```python
from build123d import *

# Parameters (mm, degrees)
SALIENTE_EXTRUIR1_DEPTH = 15
CROQUIS2_R              = 2.167600076
SALIENTE_EXTRUIR2_DEPTH = 1.2


with BuildPart() as part:
    # Croquis1 → Saliente-Extruir1 (new body)
    with BuildSketch(Plane.XY):
        Polygon((0, 0), (0, 10.369319961), (14.4, 10.369319961), (14.4, 0), (13.2, 0), (13.2, 8.869319961), (1.2, 8.869319961), (1.2, 0), align=None)
    extrude(amount=-SALIENTE_EXTRUIR1_DEPTH)

    # Croquis2 → Saliente-Extruir2 (add)
    # profile 1 of 2: a face of its own
    with BuildSketch(Plane.XZ):
        with BuildLine():
            ThreePointArc((20.704683633, -6.742646275), (24.235200152, -10.595528965), (20.704683633, -14.448411655))
            Line((20.704683633, -14.448411655), (14.4, -15))
            Line((14.4, -15), (14.4, -6.19105793))
            Line((14.4, -6.19105793), (20.704683633, -6.742646275))
        make_face()
        with Locations(Location((20.367600076, -10.595528965, 0), (0, 0, 270))):
            Circle(CROQUIS2_R, mode=Mode.SUBTRACT)
    # profile 2 of 2: a face of its own
    with BuildSketch(Plane.XZ):
        with BuildLine():
            Line((-6.304683633, -14.448411655), (0, -15))
            Line((0, -15), (0, -6.19105793))
            Line((0, -6.19105793), (-6.304683633, -6.742646275))
            ThreePointArc((-6.304683633, -6.742646275), (-9.835200152, -10.595528965), (-6.304683633, -14.448411655))
        make_face()
        with Locations(Location((-5.967600076, -10.595528965, 0), (0, 0, 270))):
            Circle(CROQUIS2_R, mode=Mode.SUBTRACT)
    extrude(amount=-SALIENTE_EXTRUIR2_DEPTH)


solid = part.part
```
Verification items for the finished model (mm, model axes). A direction names the side the tool comes from. Give positions to 0.01 mm unless a question says otherwise; leave off trailing zeros. Write each loop counter-clockwise with the first axis right and the second up, starting at its lowest first coordinate (ties: lowest second). Pieces come first, ordered by that corner, then holes. Notation, with made-up numbers: (58.5, 82.25) - (103.5, 82.25) arc R20 cw to (103.5, 103.25) - close; hole circle Ø11 at (54.5, 44.25). An arc over 180 degrees is marked (long way). Put each result on its own line as item: value.
Q1. Section check B-B on z = -10.25. Record the cut outline in (x, y), and give its area (3 significant figures).
Result:
outline: (-9.82, 0) - (-8.11, 0) - (-8.11, 1.2) - (-9.82, 1.2) - close; (-3.83, 0) - (1.2, 0) - (1.2, 8.87) - (13.2, 8.87) - (13.2, 0) - (18.23, 0) - (18.23, 1.2) - (14.4, 1.2) - (14.4, 10.37) - (0, 10.37) - (0, 1.2) - (-3.83, 1.2) - close; (22.51, 0) - (24.22, 0) - (24.22, 1.2) - (22.51, 1.2) - close
area: 56.2 mm2
Q2. Section check C-C on x = -5. Record the cut outline in (y, z), and give its area (3 significant figures).
Result:
outline: (0, -14.56) - (1.2, -14.56) - (1.2, -12.54) - (0, -12.54) - close; (0, -8.66) - (1.2, -8.66) - (1.2, -6.63) - (0, -6.63) - close
area: 4.87 mm2
Q3. Depth check by flat-ended pin: P1, Ø4.5, axis at x = 17.5, z = -11.5, coming from the +Y side; P2, Ø5, axis at y = 5, z = -6, coming from the -X side; P3, Ø5, axis at y = 8, z = -4.5, coming from the +X side. Enter the tip coordinate at first touch or a pass-through.
Result:
P1: y = 1.2
P2: x = 0
P3: x = 14.4
Q4. Scan lines: probe 1 along X at (y, z) = (7.25, -11.75); probe 2 along Y at (x, z) = (12, -13.25); probe 3 along X at (y, z) = (9.5, -13). Record each from-to range of solid material in increasing order. Write a range as from..to.
Result:
probe 1: 0..1.2, 13.2..14.4
probe 2: 8.87..10.37
probe 3: 0..14.4
Q5. Mould release check, pull along X, two halves, no side actions. Record for faces 5 (the face through (17.6, 0.59, -14.72)), 6 (the face through (7, 8.869, -7)), 7 (the face through (18, 0, -9)): released by +X, released by -X, zero draft, split by the parting line, or undercut.
Result:
face 5: released by +X
face 6: undercut
face 7: zero draft
Q6. Section check D-D on z = -5.5. Record the cut outline in (x, y).
Result:
outline: (0, 0) - (1.2, 0) - (1.2, 8.87) - (13.2, 8.87) - (13.2, 0) - (14.4, 0) - (14.4, 10.37) - (0, 10.37) - close
Q7. Set-up check for faces 1 (the face through (18, 1.2, -12)), 2 (the face through (-4, 1.2, -12)), 3 (the face through (1.2, 4, -7)), 4 (the face through (7, 10.369, -7)): record each of +Z, -Z, +X, -X, +Y, -Y from which the full face is reachable in a straight line by a thin tool's end or side.
Result:
face 1: +Z, -Z, +X, +Y
face 2: +Z, -Z, -X, +Y
face 3: +Z, -Z, -Y
face 4: +Z, -Z, +X, -X, +Y
Q8. Section check A-A on y = 8.5. Record the cut outline in (x, z).
Result:
outline: (0, -15) - (1.2, -15) - (1.2, 0) - (0, 0) - close; (13.2, -15) - (14.4, -15) - (14.4, 0) - (13.2, 0) - close
